```python
from build123d import *

# Parameters (mm, degrees)
F1_DEPTH = 20.6375
F2_W     = 3.945384
F2_H     = 9.525
F3_DEPTH = 11.1125
F4_R     = 1.27
F6_D     = 1.27
F6_DEPTH = 25.4


with BuildPart() as f1:
    # F0 (on Front) → F1 (new body)
    with BuildSketch(Plane.XZ):
        Polygon((1.972692, 4.7625), (-1.972692, 4.7625), (-4.7625, 1.972692), (-4.7625, -1.972692), (-1.972692, -4.7625), (1.972692, -4.7625), (4.7625, -1.972692), (4.7625, 1.972692), align=None)
    extrude(amount=F1_DEPTH)

    # F2 (on face) → F3 (join)
    with BuildSketch(Plane(origin=(0, 0, 0), x_dir=(-1, 0, 0), z_dir=(0, 1, 0))):
        Rectangle(F2_W, F2_H)
    extrude(amount=F3_DEPTH)

    # F4
    f4_edges = [f1.edges().sort_by_distance(p)[0] for p in [
        (0, 11.1125, 4.7625),
        (0, 11.1125, -4.7625),
    ]]
    fillet(f4_edges, radius=F4_R)

    # F6
    with Locations(Plane.YZ.offset(1.972692)):
        with Locations((6.35, 0)):
            Hole(F6_D / 2, depth=F6_DEPTH)


solid = f1.part
```
Geometry: final body of the model. Coordinates: model frame, mm. A direction names the side the tool comes from. Round coordinates to 2 decimals unless told otherwise and drop trailing zeros. Write each loop counter-clockwise with the first axis right and the second up, starting at its lowest first coordinate (ties: lowest second). Pieces come first, ordered by that corner, then holes. Notation, with made-up numbers: (63, 37) -> (85, 37) arc R19 cw to (85, 45) -> close; hole circle Ø2 at (11, 88). An arc over 180 degrees is marked (long way). Use CSV: the item, a comma, the result in double quotes. Start each with the question number.
Q1. Section D-D (y = -8.5). Return loops of the section in (x, z).
Q2. Pull-direction query (Y, two-part tool) for faces 4 (the face through (0, -20.638, 0)), 5 (the face through (-3.387, -10.174, -3.348)), 6 (the face through (-0.03, 10.73, 4.4)), 7 (the face through (-0.028, 6.984, 0.028)); classes: pulls with the +Y half, pulls with the -Y half, needs draft (parallel to the pull), parting line crosses it, or undercut.
Q3. Line query: L1, parallel to Y at x = -2.5, z = 1.25; L2, parallel to X at y = 5, z = -3.5; L3, parallel to Z at x = -0.75, y = 6.5. Output: solid intervals per line, ascending.
Q4. Section A-A (z = 0). Return loops of the section in (x, y) (1 decimal).
Q5. First-contact query: pin 1 Ø1.5 at (y, z) = (6.35, 0) entering from -X; pin 2 Ø0.8 at (x, z) = (3, 1.5) entering from +Y; pin 3 Ø4 at (y, z) = (-5, 3.5) entering from +X. Flat tips, straight axial feed; report the tip coordinate or a pass-through.
Q6. Reachability of faces 1 (the face through (3, 0, 0)), 2 (the face through (-4.762, -10, 0)), 3 (the face through (-1.973, 5, 0)) from +Z, -Z, +X, -X, +Y, -Y: full face, straight path, thin tool, end or side. Return the list, or none.
Q7. Section B-B (y = 6.35). Return loops of the section in (x, z) (1 decimal).
Q8. Section C-C (z = 1.5). Return loops of the section in (x, y).
Result sheet:
1,outline,"(-4.76, -1.97) -> (-1.97, -4.76) -> (1.97, -4.76) -> (4.76, -1.97) -> (4.76, 1.97) -> (1.97, 4.76) -> (-1.97, 4.76) -> (-4.76, 1.97) -> close"
2,face 4,"pulls with the -Y half"
2,face 5,"needs draft"
2,face 6,"pulls with the +Y half"
2,face 7,"undercut"
3,L1,"-20.64 to 0"
3,L2,"-1.97 to 1.97"
3,L3,"-4.76 to -0.62, 0.62 to 4.76"
4,outline,"(-4.8, -20.6) -> (4.8, -20.6) -> (4.8, 0) -> (2, 0) -> (2, 5.7) -> (-2, 5.7) -> (-2, 0) -> (-4.8, 0) -> close; (-2, 7) -> (2, 7) -> (2, 11.1) -> (-2, 11.1) -> close"
5,pin 1,"x = -1.97"
5,pin 2,"y = 0"
5,pin 3,"x = 4.76"
6,face 1,"+Z, -Z, +X, +Y"
6,face 2,"+Z, -Z, -X, +Y, -Y"
6,face 3,"+Z, -Z, -X, +Y"
7,outline,"(-2, -4.8) -> (2, -4.8) -> (2, -0.6) -> (-2, -0.6) -> close; (-2, 0.6) -> (2, 0.6) -> (2, 4.8) -> (-2, 4.8) -> close"
8,outline,"(-4.76, -20.64) -> (4.76, -20.64) -> (4.76, 0) -> (1.97, 0) -> (1.97, 11.11) -> (-1.97, 11.11) -> (-1.97, 0) -> (-4.76, 0) -> close"
